Could you check a few things on this model? Use its own coordinates, in mm. A direction names the side the tool comes from. Round coordinates to 2 decimals unless told otherwise and drop trailing zeros. Write each loop counter-clockwise with the first axis right and the second up, starting at its lowest first coordinate (ties: lowest second). Pieces come first, ordered by that corner, then holes. Notation, with made-up numbers: (-16.5, 0.25) - (28.5, 0.25) arc R20 cw to (28.5, 4.25) - close; hole circle Ø11 at (11.25, 57). An arc over 180 degrees is marked (long way). Put each result on its own line as item: value.
Autodesk Inventor part; units mm, degrees
ref_plane "YZ Plane" through (0, 0, 0) normal (1, 0, 0) x (0, 1, 0)
ref_plane "XZ Plane" through (0, 0, 0) normal (0, 1, 0) x (-1, 0, 0)
ref_plane "XY Plane" through (0, 0, 0) normal (0, 0, 1) x (1, 0, 0)
sketch "Sketch1" plane through (0, 0, 0) normal (0, 1, 0) x (-1, 0, 0)
  line L0 (-4.5, -21) -> (4.5, -21)
  line L1 (4.5, -21) -> (4.5, 21) construction
  line L2 (4.5, 21) -> (-4.5, 21)
  line L3 (-4.5, 21) -> (-4.5, -21)
  line L4 (-4.5, -21) -> (4.5, 21) construction
  line L5 (4.5, -21) -> (-4.5, 21) construction
  circle A0 centre (0.5, 15.5) radius 1.5
  circle A1 centre (0.5, -15.5) radius 1.5
  line L6 (0.5, 15.5) -> (0.5, -15.5) construction
  line L7 (4.5, 0) -> (0.5, 0) construction
  line L8 (6, 20) -> (-1.5, 20)
  line L9 (-1.5, 20) -> (-1.5, -20)
  line L10 (-1.5, -20) -> (6, -20)
  circle A2 centre (0.5, 15.5) radius 3
  circle A3 centre (0.5, -15.5) radius 3
  line L11 (4.5, -21) -> (6, -21)
  line L12 (6, -21) -> (6, 21)
  line L13 (6, 21) -> (4.5, 21)
  point P0 (0, 0)
  point P1 (-1.5, 0)
  point P2 (-1.5, 17.7361)
  point P3 (-1.5, 13.2639)
  point P4 (-1.5, -13.2639)
  point P5 (-1.5, -17.7361)
  dimension "d0" = 42
  dimension "d1" = 9
  dimension "d2" = 3
  dimension "d3" = 4
  dimension "d4" = 31
  dimension "d7" = 40
  dimension "d8" = 6
  dimension "d18" = 1.5
  dimension "d19" = 1.5
  dimension "d24" = 1.5
extrude "Extrusion1" add sketch "Sketch1" along normal blind 6
extrude "Extrusion2" add sketch "Sketch1" along normal blind 8 from surface at 6 contours L10 L9 A3 A2 L8 L12
sketch "Sketch3" plane through (1.5, 6, 20) normal (1, 0, 0) x (0, 0, -1)
  line L0 (2.2639, 8) -> (0, 8)
  line L1 (0, 0) -> (0, 8)
  line L2 (40, 0) -> (37.7361, 0)
  line L3 (40, 0) -> (40, 8)
  line L4 (10, 4) -> (30, 4) construction
  line L5 (37, 0) -> (37, -6) construction
  line L6 (20, 4) -> (20, 8) construction
  line L7 (40, 8) -> (0, 8) construction
  circle A0 centre (10, 4) radius 2
  circle A1 centre (30, 4) radius 2
  circle A2 centre (10, 4) radius 4
  circle A3 centre (30, 4) radius 4
  line L8 (40, 8) -> (37.7361, 8)
  line L9 (37.7361, 0) -> (37.7361, 8)
  line L10 (2.2639, 0) -> (0, 0)
  line L11 (2.2639, 0) -> (2.2639, 8)
  line L12 (33.2639, 8) -> (6.7361, 8)
  line L13 (6.7361, 0) -> (6.7361, 8)
  line L14 (33.2639, 0) -> (6.7361, 0)
  line L15 (33.2639, 0) -> (33.2639, 8)
  point P0 (20, -6)
  dimension "d11" = 20
  dimension "d12" = 4
  dimension "d15" = 4
  dimension "d22" = 8
extrude "Extrusion4" add sketch "Sketch1" along normal blind 8 from surface at 0 contours A3 L9 | L9 A3 | A2 L9 | L9 A2
extrude "Extrusion3" cut sketch "Sketch3" against normal through all contours A0 | A1
equation "\"d18\" = d19"
properties part number "Z Axis Stepper Bracket"
(1) Imagine slicing it at D-D, the plane x = -4.75. List the corners of the cut face in (y, z) for me, then the cut area to 3 significant figures.
Values found:
outline: (0, -21) - (6, -21) - (6, -20) - (14, -20) - (14, 20) - (6, 20) - (6, 21) - (0, 21) - close; hole circle Ø4 at (10, -10); hole circle Ø4 at (10, 10)
area: 547 mm^2
(2) If we mould it in two halves opening along X, with no side actions, what happens to faces 1 (the face through (3, 6, 0)), 2 (the face through (1.5, 10, 0)), 3 (the face through (-2, 8, -17))? For each: pulls with the +X half, pulls with the -X half, needs draft (parallel to the pull), parting line crosses it, or undercut.
Values found:
face 1: needs draft
face 2: pulls with the +X half
face 3: undercut
(3) I'm going to push flat-ended pins straight in: pin 1 (2 mm diameter, centred on x = -1.5, y = 10, fed in from -Z); pin 2 (1.8 mm diameter, centred on y = 9.5, z = -18.5, fed in from +X); pin 3 (3 mm diameter, centred on x = 0, z = 16.5, fed in from +Y); pin 4 (2.5 mm diameter, centred on x = -0.5, z = -15.5, fed in from +Y). Where does each tip first touch, or does it pass through?
Values found:
pin 1: stops at z = -20
pin 2: stops at x = 1.5
pin 3: stops at y = 8
pin 4: passes through
(4) Please list where these lines run through material, in increasing order: probe 1 along Z at (x, y) = (-0.5, 1.5); probe 2 along Z at (x, y) = (-0.5, 9.6); probe 3 along Z at (x, y) = (-4, 8.5). Write a range as from..to.
Values found:
probe 1: z = -21..-17, -14..14, 17..21
probe 2: z = -20..-18.5, -12.5..-11.96, -8.04..8.04, 11.96..12.5, 18.5..20
probe 3: z = -20..-11.32, -8.68..8.68, 11.32..20
(5) Imagine slicing it at C-C, the plane y = 10. List the corners of the cut face in (x, z) for me, then the cut area to 3 significant figures.
Values found:
outline: (-6, -20) - (1.5, -20) - (1.5, -17.74) arc R3 cw (long way) to (1.5, -13.26) - (1.5, -12) - (-6, -12) - close; (-6, -8) - (1.5, -8) - (1.5, 8) - (-6, 8) - close; (-6, 12) - (1.5, 12) - (1.5, 13.26) arc R3 cw (long way) to (1.5, 17.74) - (1.5, 20) - (-6, 20) - close
area: 190 mm^2
(6) Imagine slicing it at B-B, the plane x = -0.5. List the corners of the cut face in (y, z) for me.
Values found:
outline: (0, -21) - (6, -21) - (6, -20) - (14, -20) - (14, -18.5) - (8, -18.5) - (8, -17) - (0, -17) - close; (0, -14) - (8, -14) - (8, -12.5) - (14, -12.5) - (14, 12.5) - (8, 12.5) - (8, 14) - (0, 14) - close; (0, 17) - (8, 17) - (8, 18.5) - (14, 18.5) - (14, 20) - (6, 20) - (6, 21) - (0, 21) - close; hole circle Ø4 at (10, -10); hole circle Ø4 at (10, 10)
(7) Imagine slicing it at A-A, the plane z = -10. List the corners of the cut face in (x, y) for me.
Values found:
outline: (-6, 0) - (4.5, 0) - (4.5, 6) - (1.5, 6) - (1.5, 8) - (-6, 8) - close; (-6, 12) - (1.5, 12) - (1.5, 14) - (-6, 14) - close
(8) For faces 4 (the face through (-3.5, 11, -15.4)), 5 (the face through (-2, 10, -20)), 6 (the face through (2.5, 7, -15.5)), 7 (the face through (-2, 10, 20)), which set-ups out of +Z, -Z, +X, -X, +Y, -Y let a thin tool reach every point of the face, with its end or its side?
Values found:
face 4: +Y
face 5: -Z, +X, -X, +Y
face 6: +X, +Y
face 7: +Z, +X, -X, +Y
